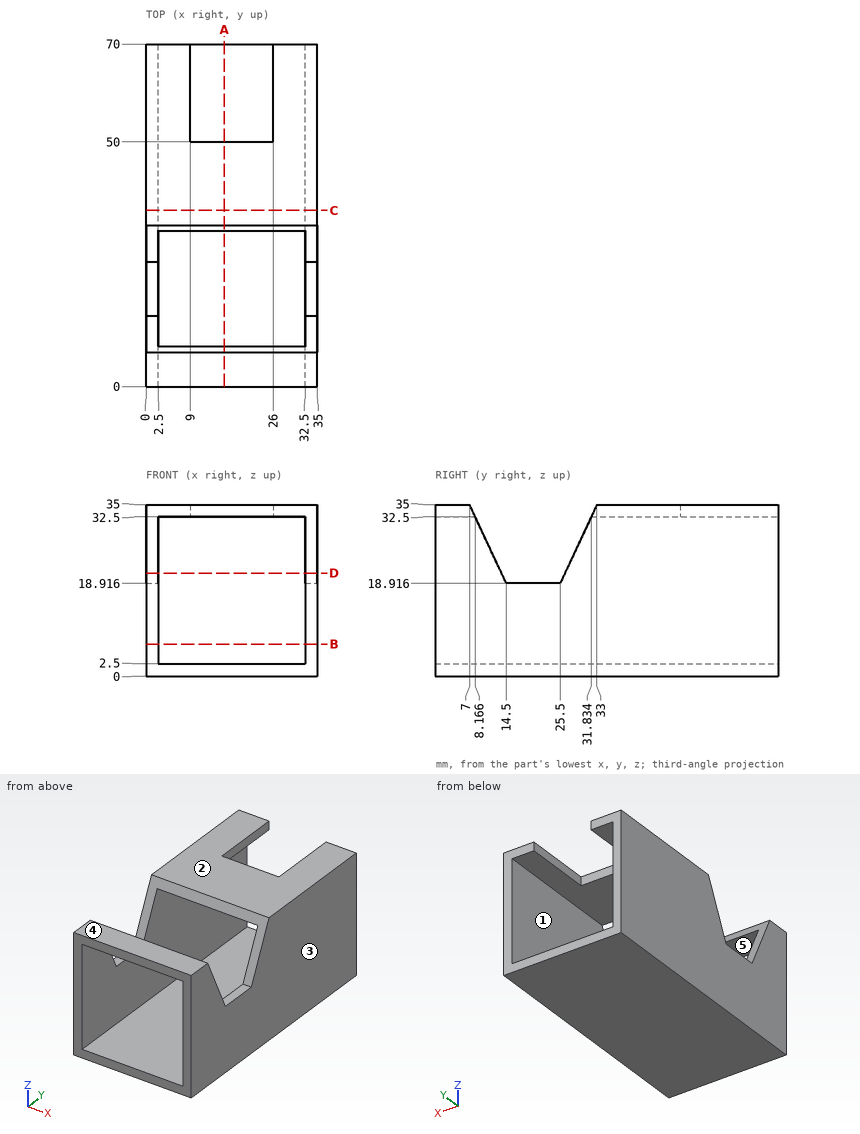
Could you check a few things on this drawing? It's one solid part, dimensions in mm from its lowest x, y, z. A direction names the side the tool comes from. Round coordinates to 2 decimals unless told otherwise and drop trailing zeros. Write each loop counter-clockwise with the first axis right and the second up, starting at its lowest first coordinate (ties: lowest second). Pieces come first, ordered by that corner, then holes.
Q1. Please list where these lines run through material, in increasing order: probe 1 along X at (y, z) = (45, 13.5); probe 2 along Z at (x, y) = (11.5, 18).
Q2. If we section it at A-A on x = 16: Write out the boundary of the cut face in (y, z).
Q3. Which directions (+Z, -Z, +X, -X, +Y, -Y) give clear straight access to the entire face, cutting with the end or side of a thin tool? Please do the marked faces 1 and 2.
Q4. If we section it at B-B on z = 6.5: Write out the boundary of the cut face in (x, y).
Q5. Will these pins go through, and if not, where does the flat tip stop? P1, Ø6, axis at y = 35, z = 20, coming from the -X side; P2, Ø8, axis at x = 9, y = 17.5, coming from the +Z side; P3, Ø1.2, axis at x = 1.5, y = 18.5, coming from the +Z side; P4, Ø1.2, axis at x = 16.5, z = 33, coming from the +Y side.
Q6. If we section it at D-D on z = 21: Write out the boundary of the cut face in (x, y), plus the area to 3 significant figures.
Q7. If we section it at C-C on y = 36: Write out the boundary of the cut face in (x, z), plus the area to 3 significant figures.
Q8. If we mould it in two halves opening along Z, with no side actions, what happens to the marked faces 3, 4 and 5? For each: +Z half, -Z half, draft (parallel to the pull), parting line (faces both ways), or undercut.
Answer below:
1. probe 1: x = 0 to 2.5, 32.5 to 35
1. probe 2: z = 0 to 2.5
2. outline: (0, 0) - (70, 0) - (70, 2.5) - (0, 2.5) - close; (0, 32.5) - (8.17, 32.5) - (7, 35) - (0, 35) - close; (31.83, 32.5) - (50, 32.5) - (50, 35) - (33, 35) - close
3. face 1: +Y, -Y
3. face 2: +Z, +X, -X, +Y, -Y
4. outline: (0, 0) - (2.5, 0) - (2.5, 70) - (0, 70) - close; (32.5, 0) - (35, 0) - (35, 70) - (32.5, 70) - close
5. P1: stops at x = 0
5. P2: stops at z = 2.5
5. P3: stops at z = 18.92
5. P4: stops at y = 50
6. outline: (0, 0) - (2.5, 0) - (2.5, 13.53) - (0, 13.53) - close; (0, 26.47) - (2.5, 26.47) - (2.5, 70) - (0, 70) - close; (32.5, 0) - (35, 0) - (35, 13.53) - (32.5, 13.53) - close; (32.5, 26.47) - (35, 26.47) - (35, 70) - (32.5, 70) - close
6. area: 285 mm2
7. outline: (0, 0) - (35, 0) - (35, 35) - (0, 35) - close; hole (2.5, 2.5) - (32.5, 2.5) - (32.5, 32.5) - (2.5, 32.5) - close
7. area: 325 mm2
8. face 3: draft
8. face 4: +Z half
8. face 5: undercut
